```python
from build123d import *

# Parameters (mm, degrees)
SKETCH1_W           = 170
SKETCH1_H           = 70
SKETCH1_W_2         = 150
SKETCH1_H_2         = 50
BOSS_EXTRUDE1_DEPTH = 80
SKETCH2_W           = 10
SKETCH2_H           = 13
BOSS_EXTRUDE2_DEPTH = 15
SKETCH3_R           = 2.381541705
CUT_EXTRUDE1_DEPTH  = 15


with BuildPart() as part:
    # Sketch1 → Boss-Extrude1 (new body)
    with BuildSketch(Plane.XY):
        Rectangle(SKETCH1_W, SKETCH1_H)
        Rectangle(SKETCH1_W_2, SKETCH1_H_2, mode=Mode.SUBTRACT)
    extrude(amount=BOSS_EXTRUDE1_DEPTH)

    # Sketch2 → Boss-Extrude2 (add)
    with BuildSketch(Plane.ZY.offset(-75)):
        with Locations((5, 18.5)):
            Rectangle(SKETCH2_W, SKETCH2_H)
    boss_extrude2 = extrude(amount=BOSS_EXTRUDE2_DEPTH)

    # Sketch3 → Cut-Extrude1 (cut)
    with BuildSketch(Plane(origin=(0, 0, 0), x_dir=(-1, 0, 0), z_dir=(0, 0, -1))):
        with Locations((-69.43110047, 20.059908975)):
            Circle(SKETCH3_R)
    cut_extrude1 = extrude(amount=-CUT_EXTRUDE1_DEPTH, mode=Mode.SUBTRACT)

    # Mirror1: Boss-Extrude2, Cut-Extrude1 across plane
    add(boss_extrude2.mirror(Plane(origin=(0, 0, 0), x_dir=(0, 0, 1), z_dir=(1, 0, 0))))
    add(cut_extrude1.mirror(Plane(origin=(0, 0, 0), x_dir=(0, 0, 1), z_dir=(1, 0, 0))), mode=Mode.SUBTRACT)


solid = part.part
```
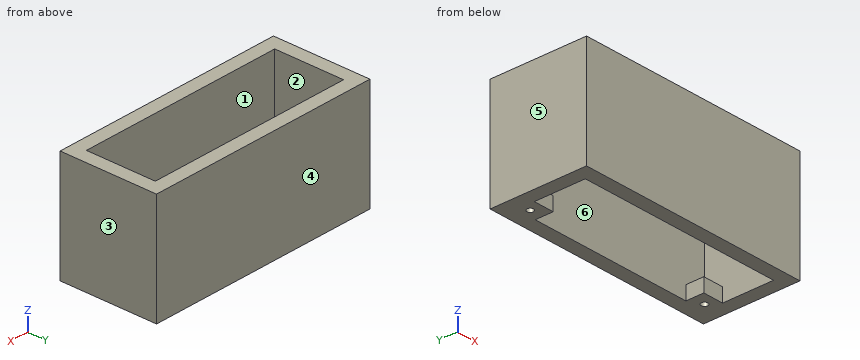
Can you work these out from the model? Positions are in its coordinate system, mm. Face numbers are marked on the shaded views. A direction names the side the tool comes from. Round coordinates to 2 decimals unless told otherwise and drop trailing zeros. Loops run counter-clockwise (first coordinate to the right, second up) from the corner with the lowest first, then second, coordinate; pieces in that order, holes last. Notation, with made-up numbers: (54.5, 48.5) -> (60.5, 48.5) arc R28 ccw to (60.5, 69.5) -> close; hole circle Ø10 at (63.5, 73). An arc over 180 degrees is marked (long way). One line per item, written item: value. Start each with the question number.
1. For pin 1 (4 mm diameter, centred on x = -64.5, y = 19.5, fed in from +Z); pin 2 (10.5 mm diameter, centred on x = 71, y = 17.5, fed in from +Z); pin 3 (3 mm diameter, centred on x = -69.43, y = 20.06, fed in from +Z), each with a flat end and sliding along its axis, tell me the tip position at first contact or that it passes through.
2. If we section it at D-D, the plane z = 7.5: Write out the boundary of the cut face in (x, y), then the cut area to 3 significant figures.
3. For the marked faces 1, 2 and 3, which set-ups out of +Z, -Z, +X, -X, +Y, -Y let a thin tool reach every point of the face, with its end or its side?
4. If we section it at A-A, the plane x = 30.5: Write out the boundary of the cut face in (y, z), then the cut area to 3 significant figures.
5. If we mould it in two halves opening along X, with no side actions, what happens to the marked faces 4, 5 and 6? For each: pulls with the +X half, pulls with the -X half, needs draft (parallel to the pull), parting line crosses it, or undercut.
6. If we section it at C-C, the plane z = 37: Write out the boundary of the cut face in (x, y), then the cut area to 3 significant figures.
7. If we section it at B-B, the plane y = -7: Write out the boundary of the cut face in (x, z).
8. If I drill on probe 1 along Y at (x, z) = (61, 7); probe 2 along Y at (x, z) = (-62.5, 40); probe 3 along X at (y, z) = (7.5, 39), over which ranges is the centre line in solid material (lowest first)?
Calculated:
1. pin 1: stops at z = 10
1. pin 2: stops at z = 80
1. pin 3: passes through
2. outline: (-85, -35) -> (85, -35) -> (85, 35) -> (-85, 35) -> close; hole (-75, -25) -> (75, -25) -> (75, 12) -> (60, 12) -> (60, 25) -> (-60, 25) -> (-60, 12) -> (-75, 12) -> close; hole circle Ø4.76 at (-69.43, 20.06); hole circle Ø4.76 at (69.43, 20.06)
2. area: 4,750 mm²
3. face 1: +Z, -Z
3. face 2: +Z
3. face 3: +Z, -Z, +X, +Y, -Y
4. outline: (-35, 0) -> (-25, 0) -> (-25, 80) -> (-35, 80) -> close; (25, 0) -> (35, 0) -> (35, 80) -> (25, 80) -> close
4. area: 1,600 mm²
5. face 4: needs draft
5. face 5: pulls with the -X half
5. face 6: undercut
6. outline: (-85, -35) -> (85, -35) -> (85, 35) -> (-85, 35) -> close; hole (-75, -25) -> (75, -25) -> (75, 25) -> (-75, 25) -> close
6. area: 4,400 mm²
7. outline: (-85, 0) -> (-75, 0) -> (-75, 80) -> (-85, 80) -> close; (75, 0) -> (85, 0) -> (85, 80) -> (75, 80) -> close
8. probe 1: y = -35 to -25, 12 to 35
8. probe 2: y = -35 to -25, 25 to 35
8. probe 3: x = -85 to -75, 75 to 85
